```python
from build123d import *


with BuildPart() as part:
    # Sketch1 → Revolve1 (revolve)
    with BuildSketch(Plane.XY, mode=Mode.PRIVATE) as revolve1_sk:
        Polygon((-99.147058824, 0), (-99.147058824, 4), (-79.147058824, 4), (-79.147058824, 5), (60.852941176, 5), (60.852941176, 7.5), (95.852941176, 20), (105.852941176, 20), (105.852941176, 10), (110.852941176, 10), (110.852941176, 5), (135.852941176, 5), (135.852941176, 4), (143.852941176, 4), (143.852941176, 3), (150.852941176, 3), (150.852941176, 0), align=None)
    revolve(revolve1_sk.sketch.rotate(Axis((-132.617647059, 0, 0), (1, 0, 0)), 90), axis=Axis((-132.617647059, 0, 0), (1, 0, 0)))  # turned: the seam where the file's is


solid = part.part
```
Here's how the part is built. I have some questions about the finished solid (model axes, mm). A direction names the side the tool comes from. Round coordinates to 2 decimals unless told otherwise and drop trailing zeros. Loops run counter-clockwise (first coordinate to the right, second up) from the corner with the lowest first, then second, coordinate; pieces in that order, holes last.
1. For faces 1 (the face through (-89.007, 3.905, -0.867)), 2 (the face through (100.92, -0.88, -19.98)), 3 (the face through (108, 0, -10)), which set-ups out of +Z, -Z, +X, -X, +Y, -Y let a thin tool reach every point of the face, with its end or its side?
Answers:
face 1: -X
face 2: +X, -X
face 3: +X
2. Suppose I cut it at D-D, the plane x = -16. Please give me the cut outline in (y, z).
Answers:
outline: circle Ø10 at (0, 0)
3. If I drill on probe 1 along Y at (x, z) = (-11.5, 4); probe 2 along Z at (x, y) = (-38, -3); probe 3 along Z at (x, y) = (115, 4.5), over which ranges is the centre line in solid material (lowest first)?
Answers:
probe 1: y = -3 to 3
probe 2: z = -4 to 4
probe 3: z = -2.18 to 2.18
4. Suppose I cut it at C-C, the plane x = -82.5. Please give me the cut outline in (y, z).
Answers:
outline: circle Ø8 at (0, 0)
5. Will these pins go through, and if not, where does the flat tip stop? pin 1 (2 mm diameter, centred on x = -37, z = 5.5, fed in from -Y); pin 2 (10 mm diameter, centred on y = -3.5, z = -0.5, fed in from +X); pin 3 (8 mm diameter, centred on y = 5.5, z = 16, fed in from +X); pin 4 (4 mm diameter, centred on x = -42, y = -0.5, fed in from +Z).
Answers:
pin 1: stops at y = -2.18
pin 2: stops at x = 150.85
pin 3: stops at x = 105.85
pin 4: stops at z = 5
